from build123d import *

# Parameters (mm, degrees)
F0_W        = 87
F0_H        = 3
F0_W_2      = 85
F0_H_2      = 1.5
F1_DEPTH    = 54.5
F3_DEPTH    = 10
F4_T1_DEPTH = 18.6923881554
F5_T1_DEPTH = 18.69
F6_W        = 87
F6_H        = 3
F7_DEPTH    = 1.2
F8_R        = 5


# Not quite as in the source:
# - a fillet or chamfer that OpenCascade refuses, or shapes differently, is made with other operations: its cross-section is extruded or revolved along the edge and cut away or added


with BuildPart() as f1:
    # F0 (on Top) → F1 (new body)
    with BuildSketch(Plane.XY):
        with Locations((18.8151740879, 14.6483827978)):
            Rectangle(F0_W, F0_H)
        with Locations((18.7021535635, 14.5136903673)):
            Rectangle(F0_W_2, F0_H_2, mode=Mode.SUBTRACT)
    extrude(amount=F1_DEPTH)

    # F2 (on face) → F3 (cut)
    with BuildSketch(Plane.XZ.offset(-13.1483827978)):
        with BuildLine():
            Line((28.1252544373, 54.5), (7.2028026916, 54.5))
            ThreePointArc((7.2028026916, 54.5), (17.6640285645, 44.8635037778), (28.1252544373, 54.5))
        make_face()
    extrude(amount=-F3_DEPTH, mode=Mode.SUBTRACT)

    # F4: fillet of radius 3.1384776311 on 1 edges, made by hand

    # F4_s2 → F4_t1 (cut)
    with BuildSketch(Plane.XZ.offset(-23.9945768755)):
        with BuildLine():
            ThreePointArc((59.1766964568, 54.5), (61.3959352723, 53.5807611845), (62.3151740879, 51.3615223689))
            Line((62.3151740879, 51.3615223689), (62.3151740879, 54.5))
            Line((62.3151740879, 54.5), (59.1766964568, 54.5))
        make_face()
    extrude(amount=F4_T1_DEPTH, mode=Mode.SUBTRACT)

    # F5: fillet of radius 3.138 on 1 edges, made by hand

    # F5_s2 → F5_t1 (cut)
    with BuildSketch(Plane.XZ.offset(-23.9933827978)):
        with BuildLine():
            ThreePointArc((-24.6848259121, 51.362), (-23.7657269915, 53.5809010794), (-21.5468259121, 54.5))
            Line((-21.5468259121, 54.5), (-24.6848259121, 54.5))
            Line((-24.6848259121, 54.5), (-24.6848259121, 51.362))
        make_face()
    extrude(amount=F5_T1_DEPTH, mode=Mode.SUBTRACT)

    # F6 (on Top) → F7 (join)
    with BuildSketch(Plane.XY):
        with Locations((18.8151740879, 14.6483827978)):
            Rectangle(F6_W, F6_H)
    extrude(amount=-F7_DEPTH)

    # F8
    f8_edges = [f1.edges().sort_by_distance(p)[0] for p in [
        (28.125254, 13.456037, 54.5),
        (28.125254, 15.706037, 54.5),
        (7.202803, 13.456037, 54.5),
        (7.202803, 15.706037, 54.5),
    ]]
    fillet(f8_edges, radius=F8_R)


solid = f1.part
Check sheet for the modelled part. Datum: model origin and axes. Units: mm. A direction names the side the tool comes from. Coordinates: 2 decimals unless noted, no trailing zeros. Write each loop counter-clockwise with the first axis right and the second up, starting at its lowest first coordinate (ties: lowest second). Pieces come first, ordered by that corner, then holes.
Item 1: Cross-section at A-A on z = 29.5. Record the boundary of the cut face in (x, y).
Numbers:
outline: (-24.68, 13.15) - (62.32, 13.15) - (62.32, 16.15) - (-24.68, 16.15) - close; hole (-23.8, 13.76) - (61.2, 13.76) - (61.2, 15.26) - (-23.8, 15.26) - close
Item 2: Scan lines: probe 1 along Y at (x, z) = (-7, 5); probe 2 along X at (y, z) = (15.1, 10); probe 3 along Z at (x, y) = (18.5, 15.1). Record each from-to range of solid material in increasing order.
Numbers:
probe 1: y = 13.15 to 13.76, 15.26 to 16.15
probe 2: x = -24.68 to -23.8, 61.2 to 62.32
probe 3: z = -1.2 to 0
Item 3: Cross-section at B-B on x = -9.5. Record the boundary of the cut face in (y, z).
Numbers:
outline: (13.15, -1.2) - (16.15, -1.2) - (16.15, 54.5) - (15.26, 54.5) - (15.26, 0) - (13.76, 0) - (13.76, 54.5) - (13.15, 54.5) - close
Item 4: Access from +Z, -Z, +X, -X, +Y, -Y to the whole of each face (thin tool, end or side, straight path). Record for faces 4 (the face through (6.14, 15.71, 53.63)), 5 (the face through (-24.685, 15, 25)), 6 (the face through (18, 15.264, 27)).
Numbers:
face 4: +Z, +Y, -Y
face 5: +Z, -Z, -X, +Y, -Y
face 6: +Z
Item 5: Cross-section at C-C on y = 14.7. Record the boundary of the cut face in (x, z).
Numbers:
outline: (-24.68, -1.2) - (62.32, -1.2) - (62.32, 51.36) arc R3.14 ccw to (61.2, 53.76) - (61.2, 0) - (-23.8, 0) - (-23.8, 53.55) arc R3.14 ccw to (-24.68, 51.36) - close
Item 6: Cross-section at D-D on z = 48. Record the boundary of the cut face in (x, y), then the cut area to 3 significant figures.
Numbers:
outline: (-24.68, 13.15) - (10.18, 13.15) - (10.18, 13.76) - (-23.8, 13.76) - (-23.8, 15.26) - (10.18, 15.26) - (10.18, 16.15) - (-24.68, 16.15) - close; (25.15, 13.15) - (62.32, 13.15) - (62.32, 16.15) - (25.15, 16.15) - (25.15, 15.26) - (61.2, 15.26) - (61.2, 13.76) - (25.15, 13.76) - close
area: 111 mm2
Item 7: Mould release check, pull along X, two halves, no side actions. Record for faces 1 (the face through (-24.14, 14.67, 53.13)), 2 (the face through (18, 16.148, 27)), 3 (the face through (29.3, 15.7, 53.7)): released by +X, released by -X, zero draft, split by the parting line, or undercut.
Numbers:
face 1: released by -X
face 2: zero draft
face 3: undercut
